Geometry: see drawing. Coordinates: mm, zero at the bounding-box minimum. Coordinates: 2 decimals unless noted, no trailing zeros. Order: outer loops, then holes, each group sorted by start corner. A loop starts at its lowest first (then second) coordinate and runs counter-clockwise, first axis right, second up. Notation, with made-up numbers: (3, 86) - (56, 86) arc R10 ccw to (56, 95) - close; hole circle Ø11 at (-36, 0.25). An arc over 180 degrees is marked (long way). Use a Markdown table: item, result. Add a question column.
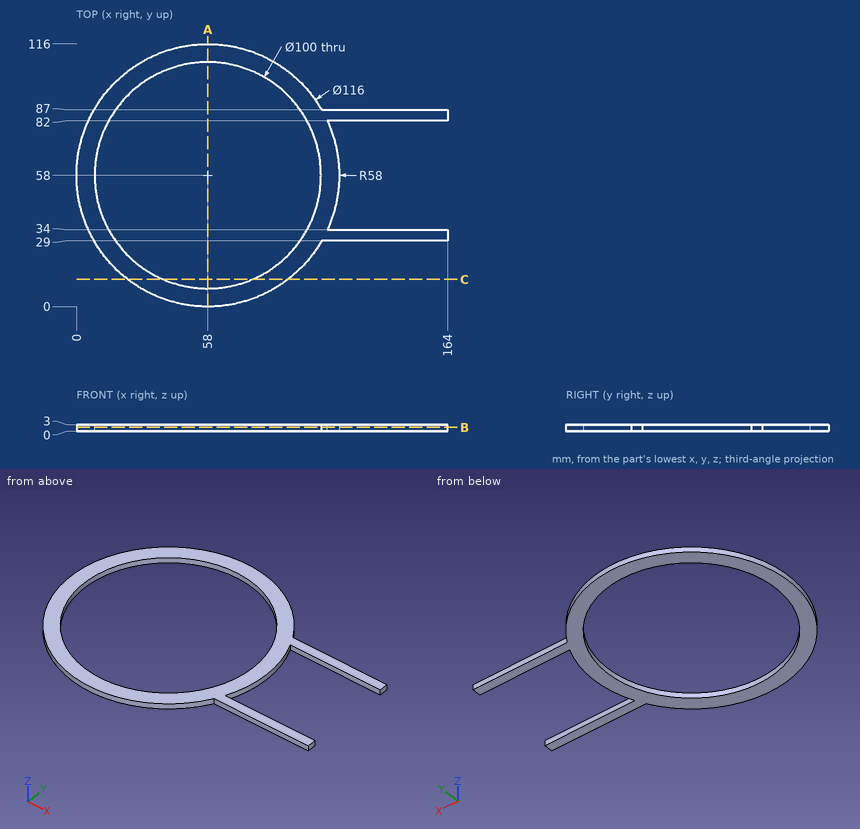
1) Cut plane C-C (y = 12). Return the cut outline in (x, z), and give its area (3 significant figures).
2) Cut plane A-A (x = 58). Return the cut outline in (y, z), and give its area (3 significant figures).
3) Material intervals for L1, parallel to Y at x = 134, z = 1.5; L2, parallel to X at y = 58, z = 2.05, sorted ascending.
4) Contact query for flat-ended pins moving along their axis: P1, Ø1.5, axis at x = 97.5, z = 1, coming from the -Y side; P2, Ø0.9, axis at x = 124.5, z = 2, coming from the +Y side; P3, Ø1.5, axis at x = 133.5, z = 2, coming from the -Y side. Output: stop coordinate, or through.
5) Cut plane B-B (z = 1.85). Return the cut outline in (x, y).
Computed:
| question | item | result |
|---|---|---|
| 1 | outline | (22.67, 0) - (38.4, 0) - (38.4, 3) - (22.67, 3) - close; (77.6, 0) - (93.33, 0) - (93.33, 3) - (77.6, 3) - close |
| 1 | area | 94.4 mm2 |
| 2 | outline | (0, 0) - (8, 0) - (8, 3) - (0, 3) - close; (108, 0) - (116, 0) - (116, 3) - (108, 3) - close |
| 2 | area | 48.0 mm2 |
| 3 | L1 | y = 29 to 34, 82 to 87 |
| 3 | L2 | x = 0 to 8, 108 to 116 |
| 4 | P1 | stops at y = 14.84 |
| 4 | P2 | stops at y = 87 |
| 4 | P3 | stops at y = 29 |
| 5 | outline | (108.23, 29) - (164, 29) - (164, 34) - (110.8, 34) arc R58 ccw to (110.8, 82) - (164, 82) - (164, 87) - (108.23, 87) arc R58 ccw (long way) to start; hole circle Ø100 at (58, 58) |
